from build123d import *

# Parameters (mm, degrees)
BOSS_EXTRUDE1_DEPTH     = 3
SKETCH2_R               = 1.5
CUT_EXTRUDE1_DEPTH      = 65.778468645
SKETCH3_R               = 1.5
CUT_EXTRUDE2_DEPTH      = 65.778468645
SKETCH4_R               = 1.5
CUT_EXTRUDE3_DEPTH      = 65.778468645
SKETCH5_W               = 90
SKETCH5_H               = 22.75
CUT_EXTRUDE4_DEPTH      = 65.778468645
CUT_EXTRUDE5_DEPTH      = 65.778468645
CUT_EXTRUDE5_DEPTH_BACK = 65.778468645
SKETCH6_R               = 1.5
SKETCH7_R               = 1.5
CUT_EXTRUDE6_DEPTH      = 65.778468645
SKETCH8_R               = 1.5
CUT_EXTRUDE7_DEPTH      = 65.778468645
SKETCH9_R               = 1.5
CUT_EXTRUDE8_DEPTH      = 65.778468645


with BuildPart() as part:
    # Sketch1 → Boss-Extrude1 (new body)
    with BuildSketch(Plane(origin=(0, 0, 0), x_dir=(1, 0, 0), z_dir=(0, 1, 0))):
        Polygon((-45, 46.5), (-45, -46.5), (15, -46.5), (15, -1), (26, -1), (26, -46.5), (45, -46.5), (45, 46.5), align=None)
    extrude(amount=BOSS_EXTRUDE1_DEPTH)

    # Sketch2 → Cut-Extrude1 (cut, through all)
    with BuildSketch(Plane(origin=(0, 3, 0), x_dir=(1, 0, 0), z_dir=(0, 1, 0))):
        with Locations(Location((39, 4.5, 0), (0, 0, 270))):
            Circle(SKETCH2_R)
        with Locations(Location((39, -10.5, 0), (0, 0, 270))):
            Circle(SKETCH2_R)
        with Locations(Location((-39, 4.5, 0), (0, 0, 270))):
            Circle(SKETCH2_R)
        with Locations(Location((-39, -10.5, 0), (0, 0, 270))):
            Circle(SKETCH2_R)
    extrude(amount=-CUT_EXTRUDE1_DEPTH, mode=Mode.SUBTRACT)

    # Sketch3 → Cut-Extrude2 (cut, through all)
    with BuildSketch(Plane(origin=(0, 3, 0), x_dir=(1, 0, 0), z_dir=(0, 1, 0))):
        with Locations(Location((29, -20.75, 0), (0, 0, 270))):
            Circle(SKETCH3_R)
        with Locations(Location((12, -20.75, 0), (0, 0, 270))):
            Circle(SKETCH3_R)
    extrude(amount=-CUT_EXTRUDE2_DEPTH, mode=Mode.SUBTRACT)

    # Sketch4 → Cut-Extrude3 (cut, through all)
    with BuildSketch(Plane(origin=(0, 3, 0), x_dir=(1, 0, 0), z_dir=(0, 1, 0))):
        with Locations(Location((12, -9.25, 0), (0, 0, 270))):
            Circle(SKETCH4_R)
        with Locations(Location((29, -9.25, 0), (0, 0, 270))):
            Circle(SKETCH4_R)
    extrude(amount=-CUT_EXTRUDE3_DEPTH, mode=Mode.SUBTRACT)

    # Sketch5 → Cut-Extrude4 (cut, through all)
    with BuildSketch(Plane(origin=(0, 3, 0), x_dir=(1, 0, 0), z_dir=(0, 1, 0))):
        with Locations((0, -35.125)):
            Rectangle(SKETCH5_W, SKETCH5_H)
    extrude(amount=-CUT_EXTRUDE4_DEPTH, mode=Mode.SUBTRACT)

    # Sketch6 → Cut-Extrude5 (cut, two sides: drawn at the far end of the back side and taken through both)
    with BuildSketch(Plane(origin=(0, 3, 0), x_dir=(1, 0, 0), z_dir=(0, 1, 0)).offset(-CUT_EXTRUDE5_DEPTH_BACK)):
        with Locations(Location((20.5, 2.75, 0), (0, 0, 270))):
            Circle(SKETCH6_R)
        with Locations(Location((33, 2.75, 0), (0, 0, 270))):
            Circle(SKETCH6_R)
        with Locations(Location((8, 2.75, 0), (0, 0, 270))):
            Circle(SKETCH6_R)
    extrude(amount=CUT_EXTRUDE5_DEPTH + CUT_EXTRUDE5_DEPTH_BACK, mode=Mode.SUBTRACT)

    # Sketch7 → Cut-Extrude6 (cut, through all)
    with BuildSketch(Plane(origin=(0, 3, 0), x_dir=(1, 0, 0), z_dir=(0, 1, 0))):
        with Locations(Location((-39, 23.5, 0), (0, 0, 270))):
            Circle(SKETCH7_R)
        with Locations(Location((39, 23.5, 0), (0, 0, 270))):
            Circle(SKETCH7_R)
    extrude(amount=-CUT_EXTRUDE6_DEPTH, mode=Mode.SUBTRACT)

    # Sketch8 → Cut-Extrude7 (cut, through all)
    with BuildSketch(Plane(origin=(0, 3, 0), x_dir=(1, 0, 0), z_dir=(0, 1, 0))):
        with Locations(Location((-39, 43.5, 0), (0, 0, 270))):
            Circle(SKETCH8_R)
        with Locations(Location((39, 43.5, 0), (0, 0, 270))):
            Circle(SKETCH8_R)
    extrude(amount=-CUT_EXTRUDE7_DEPTH, mode=Mode.SUBTRACT)

    # Sketch9 → Cut-Extrude8 (cut, through all)
    with BuildSketch(Plane(origin=(0, 3, 0), x_dir=(1, 0, 0), z_dir=(0, 1, 0))):
        with Locations(Location((-20.5, 2.75, 0), (0, 0, 270))):
            Circle(SKETCH9_R)
        with Locations(Location((-20.5, 10.75, 0), (0, 0, 270))):
            Circle(SKETCH9_R)
    extrude(amount=-CUT_EXTRUDE8_DEPTH, mode=Mode.SUBTRACT)


solid = part.part
Verification items for the finished model (mm, model axes). A direction names the side the tool comes from. Coordinates: 2 decimals unless noted, no trailing zeros. Write each loop counter-clockwise with the first axis right and the second up, starting at its lowest first coordinate (ties: lowest second). Pieces come first, ordered by that corner, then holes. Notation, with made-up numbers: (-12, 4) - (-2, 4) arc R19 cw to (-2, 26) - close; hole circle Ø7 at (-33, 84.5). An arc over 180 degrees is marked (long way). Answer as a JSON object with one key per item and string values.
(1) Cross-section at C-C on y = 1.55. Give the number of separate pieces and of enclosed holes in the cut face, plus the area to 3 significant figures.
Report:
{"separate pieces": "1", "enclosed holes": "17", "area": "5,950 mm^2"}
(2) Mould release check, pull along Z, two halves, no side actions. Record for faces 3 (the cylindrical face through (-19.235, 1.521, -1.944)), 4 (the flat face through (20, 1, 1)), 5 (the flat face through (-1, 0, -12)): pulls with the +Z half, pulls with the -Z half, needs draft (parallel to the pull), parting line crosses it, or undercut.
Report:
{"face 3": "undercut", "face 4": "pulls with the +Z half", "face 5": "needs draft"}
(3) Cross-section at D-D on x = 39. Record the cut outline in (y, z), plus the area to 3 significant figures.
Report:
{"outline": "(0, -46.5) - (3, -46.5) - (3, -45) - (0, -45) - close; (0, -42) - (3, -42) - (3, -25) - (0, -25) - close; (0, -22) - (3, -22) - (3, -6) - (0, -6) - close; (0, -3) - (3, -3) - (3, 9) - (0, 9) - close; (0, 12) - (3, 12) - (3, 23.75) - (0, 23.75) - close", "area": "175 mm^2"}
(4) Cross-section at A-A on z = 17.5. Record the cut outline in (x, y), plus the area to 3 significant figures.
Report:
{"outline": "(-45, 0) - (15, 0) - (15, 3) - (-45, 3) - close; (26, 0) - (45, 0) - (45, 3) - (26, 3) - close", "area": "237 mm^2"}
(5) Thickness scan on line 1 along X through (y, z) = (2.05, -4.5); line 2 along X through (y, z) = (1.45, 20.75); line 3 along X through (y, z) = (2.6, 4.5). Record the ranges inside material, lowest first.
Report:
{"line 1": "-45 to -40.5, -37.5 to 37.5, 40.5 to 45", "line 2": "-45 to 10.5, 13.5 to 15, 26 to 27.5, 30.5 to 45", "line 3": "-45 to 15, 26 to 45"}
(6) Tool access check on faces 1 (the flat face through (26, 1, 12)), 2 (the cylindrical face through (-40.464, 1.521, 10.175)). Record the directions out of +Z, -Z, +X, -X, +Y, -Y that give a thin tool (end or side, any length) a straight path to the whole face; none if there is none.
Report:
{"face 1": "+Z, +Y, -Y", "face 2": "+Y, -Y"}
(7) Cross-section at B-B on x = -20.5. Record the cut outline in (y, z), plus the area to 3 significant figures.
Report:
{"outline": "(0, -46.5) - (3, -46.5) - (3, -12.25) - (0, -12.25) - close; (0, -9.25) - (3, -9.25) - (3, -4.25) - (0, -4.25) - close; (0, -1.25) - (3, -1.25) - (3, 23.75) - (0, 23.75) - close", "area": "193 mm^2"}
